Drawing for the job (mm, zero at the part's lowest x, y, z). A direction names the side the tool comes from. Coordinates: 2 decimals unless noted, no trailing zeros. Write each loop counter-clockwise with the first axis right and the second up, starting at its lowest first coordinate (ties: lowest second). Pieces come first, ordered by that corner, then holes. Notation, with made-up numbers: M -18,85 L -5,85 A21 ccw -5,113 Z; hole C -1,81.5 d2. An arc over 180 degrees is marked long. Put each result on its own line as item: value. Start each with the question number.
Q1. Pull direction X, two halves, no side cores. Call the marked faces 1, 2, 3 and 4: pulls with the +X half, pulls with the -X half, needs draft (parallel to the pull), parting line crosses it, or undercut.
Q2. Cut at A-A (z = 6). Write the cut outline in (x, y).
Q3. Cut at C-C (x = 7). Write the cut outline in (y, z), then the cut area to 3 significant figures.
Q4. Drill centre lines: line 1 along X through (y, z) = (5.25, 6); line 2 along Z through (x, y) = (35.5, 6.25); line 3 along X through (y, z) = (6, 6.75). Where is each one in solid material? Low to high.
Q5. Cut at B-B (y = 6). Write the cut outline in (x, z), then the cut area to 3 significant figures.
Q6. Cut at D-D (x = 34.5). Write the cut outline in (y, z), then the cut area to 3 significant figures.
Q7. Drop flat-ended pins along their axis: pin 1 (2 mm diameter, centred on x = 6.5, y = 3.5, fed in from -Z); pin 2 (5 mm diameter, centred on x = 5, z = 10, fed in from -Y); pin 3 (5 mm diameter, centred on x = 35.5, z = 6, fed in from -Y). Give the stop position or say it passes through.
Q8. Which spindle directions (+Z, -Z, +X, -X, +Y, -Y) get a long thin tool onto all of the face, cutting with end or side? Do the marked faces 5 and 6. Say none if no direction does.
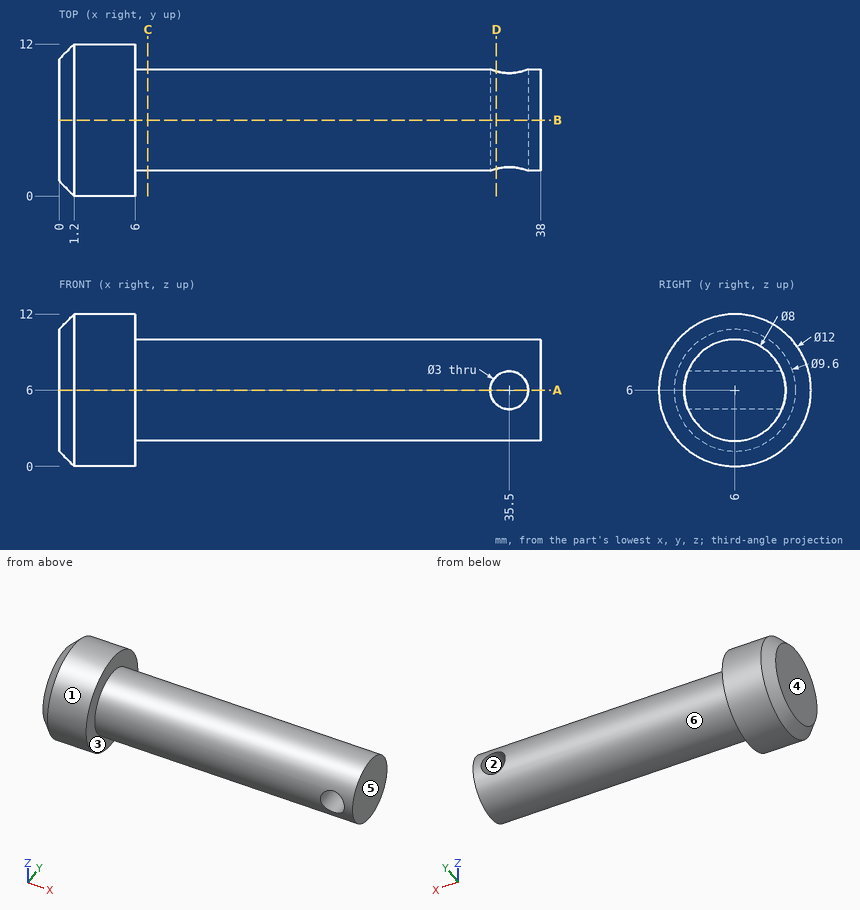
Computed values:
1. face 1: needs draft
1. face 2: undercut
1. face 3: pulls with the +X half
1. face 4: pulls with the -X half
2. outline: M 0,1.2 L 1.2,0 L 6,0 L 6,2 L 34,2 L 34,10 L 6,10 L 6,12 L 1.2,12 L 0,10.8 Z; M 37,2 L 38,2 L 38,10 L 37,10 Z
3. outline: C 6,6 d8
3. area: 50.3 mm2
4. line 1: 0 to 34, 37 to 38
4. line 2: 2.01 to 4.5, 7.5 to 9.99
4. line 3: 0 to 34.2, 36.8 to 38
5. outline: M 0,1.2 L 1.2,0 L 6,0 L 6,2 L 38,2 L 38,10 L 6,10 L 6,12 L 1.2,12 L 0,10.8 Z; hole C 35.5,6 d3
5. area: 319 mm2
6. outline: M 2.16,4.88 A4 ccw 9.84,4.88 Z; M 2.16,7.12 L 9.84,7.12 A4 ccw Z
6. area: 32.6 mm2
7. pin 1: z = 0.23
7. pin 2: y = 0.19
7. pin 3: y = 2
8. face 5: +Z, -Z, +X, +Y, -Y
8. face 6: +X
